Can you work these out from the model? Positions are in its coordinate system, mm. Give positions to 0.01 mm unless a question says otherwise; leave off trailing zeros. Order: outer loops, then holes, each group sorted by start corner. A loop starts at its lowest first (then second) coordinate and runs counter-clockwise, first axis right, second up. Notation, with made-up numbers: M -19.75,-22.5 L -4.75,-22.5 A19 ccw -4.75,14.5 Z; hole C -37,53 d6. An arc over 180 degrees is marked long. Answer as a JSON object with one key per item and string values.
```python
from build123d import *

# Parameters (mm, degrees)
BOSS_EXTRUDE2_OUTLINE_W = 304.8
BOSS_EXTRUDE2_OUTLINE_H = 50.038
BOSS_EXTRUDE2_DEPTH     = 39.99992
SKETCH3_R               = 4.7625
CUT_EXTRUDE1_DEPTH      = 312.459202856
SKETCH4_R               = 8.7376
CUT_EXTRUDE2_DEPTH      = 15.875


# Read off the part's stored shape, not the designer's step: Boss-Extrude2
with BuildPart() as part:
    # Boss-Extrude2 outline → Boss-Extrude2 (new body)
    with BuildSketch(Plane(origin=(0, 0, 0), x_dir=(1, 0, 0), z_dir=(0, 1, 0))):
        with Locations((152.4, 25.019)):
            Rectangle(BOSS_EXTRUDE2_OUTLINE_W, BOSS_EXTRUDE2_OUTLINE_H)
    extrude(amount=BOSS_EXTRUDE2_DEPTH)

    # Sketch3 → Cut-Extrude1 (cut, through all)
    with BuildSketch(Plane(origin=(0, 39.99992, 0), x_dir=(1, 0, 0), z_dir=(0, 1, 0))):
        with Locations(Location((279.4, 25.019, 0), (0, 0, 270))):
            Circle(SKETCH3_R)
        with Locations(Location((25.4, 25.019, 0), (0, 0, 270))):
            Circle(SKETCH3_R)
    extrude(amount=-CUT_EXTRUDE1_DEPTH, mode=Mode.SUBTRACT)

    # Sketch4 → Cut-Extrude2 (cut)
    with BuildSketch(Plane(origin=(0, 39.99992, 0), x_dir=(1, 0, 0), z_dir=(0, 1, 0))):
        with Locations(Location((279.4, 25.019, 0), (0, 0, 270))):
            Circle(SKETCH4_R)
        with Locations(Location((25.4, 25.019, 0), (0, 0, 270))):
            Circle(SKETCH4_R)
    extrude(amount=-CUT_EXTRUDE2_DEPTH, mode=Mode.SUBTRACT)


solid = part.part
```
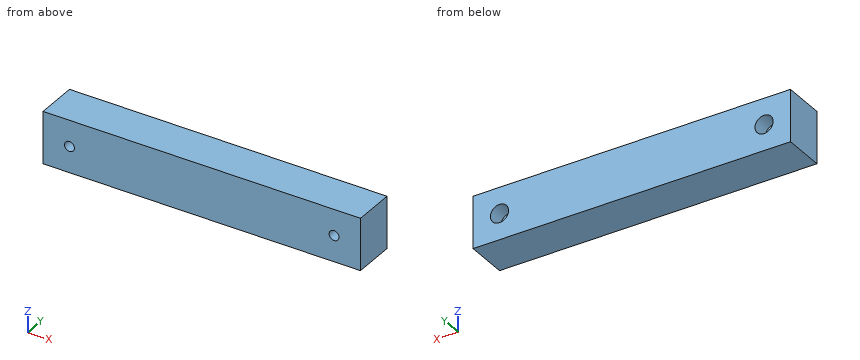
1) I need wall thicknesses on L1, parallel to X at y = 30.5, z = -21.5; L2, parallel to X at y = 33, z = -26.5; L3, parallel to Z at x = 279, y = 9. Which ranges of each line are inside material? Lowest first, please.
Results found:
{"L1": "x = 0 to 17.4, 33.4 to 271.4, 287.4 to 304.8", "L2": "x = 0 to 16.79, 34.01 to 270.79, 288.01 to 304.8", "L3": "z = -50.04 to -29.76, -20.27 to 0"}
2) I'm going to push a flat-ended pin straight in: pin 1 Ø8.5 at (x, z) = (282.5, -26) entering from +Y. Where does the tip first touch, or does it pass through?
Results found:
{"pin 1": "stops at y = 24.12"}
3) I want a section at A-A on x = 279.4. Write out the boundary of the cut face in (y, z), and give its area (3 significant figures).
Results found:
{"outline": "M 0,-50.04 L 40,-50.04 L 40,-33.76 L 24.12,-33.76 L 24.12,-29.78 L 0,-29.78 Z; M 0,-20.26 L 24.12,-20.26 L 24.12,-16.28 L 40,-16.28 L 40,0 L 0,0 Z", "area": "1,490 mm²"}
4) I want a section at B-B on y = 30. Write out the boundary of the cut face in (x, z), and give its area (3 significant figures).
Results found:
{"outline": "M 0,-50.04 L 304.8,-50.04 L 304.8,0 L 0,0 Z; hole C 25.4,-25.02 d17.48; hole C 279.4,-25.02 d17.48", "area": "14,800 mm²"}
